Here's the drawing with two shaded views (mm, measured from the low corner). I have some questions. Round coordinates to 2 decimals unless told otherwise and drop trailing zeros. Loops run counter-clockwise (first coordinate to the right, second up) from the corner with the lowest first, then second, coordinate; pieces in that order, holes last.
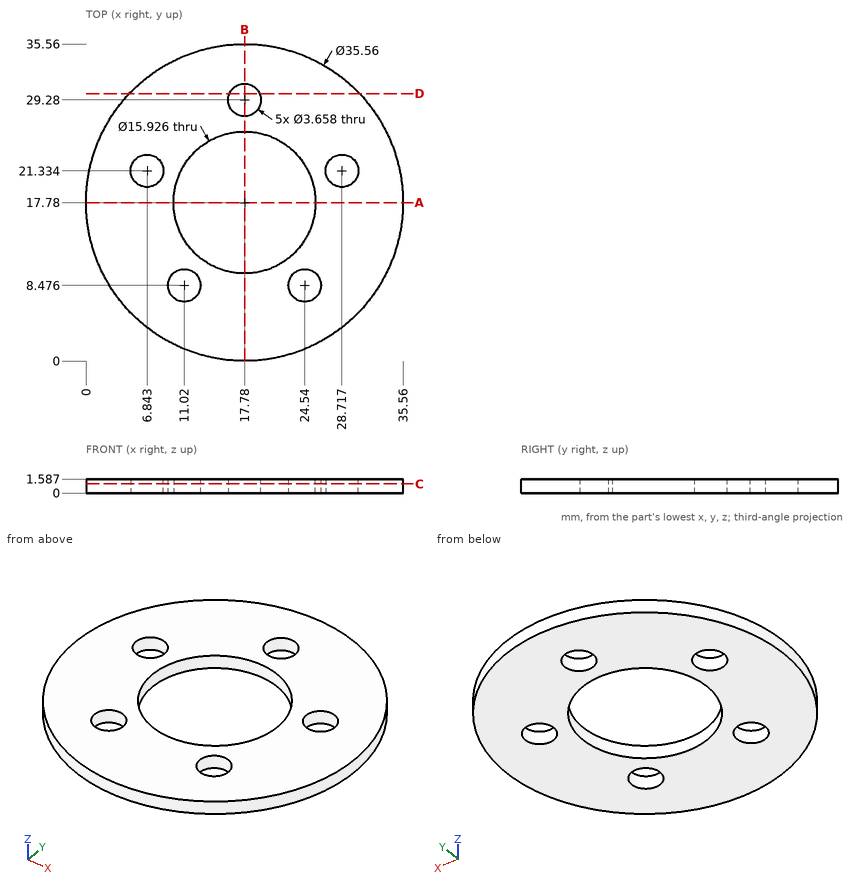
(1) If we section it at A-A, the plane y = 17.78: List the corners of the cut face in (x, z) for me.
Worked answers:
outline: (0, 0) - (9.82, 0) - (9.82, 1.59) - (0, 1.59) - close; (25.74, 0) - (35.56, 0) - (35.56, 1.59) - (25.74, 1.59) - close
(2) If we section it at B-B, the plane x = 17.78: List the corners of the cut face in (y, z) for me.
Worked answers:
outline: (0, 0) - (9.82, 0) - (9.82, 1.59) - (0, 1.59) - close; (25.74, 0) - (27.45, 0) - (27.45, 1.59) - (25.74, 1.59) - close; (31.11, 0) - (35.56, 0) - (35.56, 1.59) - (31.11, 1.59) - close
(3) If we section it at D-D, the plane y = 30: List the corners of the cut face in (x, z) for me (1 decimal).
Worked answers:
outline: (4.9, 0) - (16.1, 0) - (16.1, 1.6) - (4.9, 1.6) - close; (19.5, 0) - (30.7, 0) - (30.7, 1.6) - (19.5, 1.6) - close
(4) If I drill on line 1 (Y direction, x = 17.78, z = 0.9); line 2 (X direction, y = 8, z = 0.85) (1 decimal); line 3 (Y direction, x = 17, z = 1.5) (1 decimal), over which ranges is the centre line in solid material (lowest first)?
Worked answers:
line 1: y = 0 to 9.82, 25.74 to 27.45, 31.11 to 35.56
line 2: x = 2.9 to 9.3, 12.8 to 22.8, 26.3 to 32.6
line 3: y = 0 to 9.9, 25.7 to 27.6, 30.9 to 35.5
(5) If we section it at C-C, the plane z = 1.05: List the corners of the cut face in (x, y) for me (1 decimal).
Worked answers:
outline: circle Ø35.6 at (17.8, 17.8); hole circle Ø3.7 at (6.8, 21.3); hole circle Ø3.7 at (11, 8.5); hole circle Ø15.9 at (17.8, 17.8); hole circle Ø3.7 at (17.8, 29.3); hole circle Ø3.7 at (24.5, 8.5); hole circle Ø3.7 at (28.7, 21.3)
